CAD build for the part. Positions are in the model's coordinates, mm. Give positions to 0.01 mm unless a question says otherwise; leave off trailing zeros. Order: outer loops, then holes, each group sorted by start corner. A loop starts at its lowest first (then second) coordinate and runs counter-clockwise, first axis right, second up.
from build123d import *

# Parameters (mm, degrees)
FLOOR_MOUNT_AND_JOINT_HOLES_PROFILE_R   = 2.75
FLOOR_MOUNT_AND_JOINT_HOLES_PROFILE_R_2 = 1.75
FLOOR_MOUNT_AND_JOINT_HOLES_PROFILE_R_3 = 2.25
FLOOR_MOUNT_AND_JOINT_HOLES_PROFILE_R_4 = 2.2
FLOOR_MOUNT_AND_JOINT_HOLES_DEPTH       = 1


with BuildPart() as part:
    # Floor, mount and joint holes profile → Floor, mount and joint holes (new body)
    with BuildSketch(Plane.XY):
        Polygon((-140, -143), (-94, -143), (-94, -104), (93, -104), (93, -143), (103, -143), (103, 143), (93, 143), (93, 104), (-94, 104), (-94, 143), (-140, 143), align=None)
        with Locations((-90, -91)):
            Circle(FLOOR_MOUNT_AND_JOINT_HOLES_PROFILE_R, mode=Mode.SUBTRACT)
        with Locations((-90, 91)):
            Circle(FLOOR_MOUNT_AND_JOINT_HOLES_PROFILE_R, mode=Mode.SUBTRACT)
        with Locations((-31, -91)):
            Circle(FLOOR_MOUNT_AND_JOINT_HOLES_PROFILE_R, mode=Mode.SUBTRACT)
        with Locations((-31, 91)):
            Circle(FLOOR_MOUNT_AND_JOINT_HOLES_PROFILE_R, mode=Mode.SUBTRACT)
        with Locations((31, -91)):
            Circle(FLOOR_MOUNT_AND_JOINT_HOLES_PROFILE_R, mode=Mode.SUBTRACT)
        with Locations((31, 91)):
            Circle(FLOOR_MOUNT_AND_JOINT_HOLES_PROFILE_R, mode=Mode.SUBTRACT)
        with Locations((90, -91)):
            Circle(FLOOR_MOUNT_AND_JOINT_HOLES_PROFILE_R, mode=Mode.SUBTRACT)
        with Locations((90, 91)):
            Circle(FLOOR_MOUNT_AND_JOINT_HOLES_PROFILE_R, mode=Mode.SUBTRACT)
        with Locations((-136.5, -108)):
            Circle(FLOOR_MOUNT_AND_JOINT_HOLES_PROFILE_R_2, mode=Mode.SUBTRACT)
        with Locations((-136.5, -17)):
            Circle(FLOOR_MOUNT_AND_JOINT_HOLES_PROFILE_R_2, mode=Mode.SUBTRACT)
        with Locations((-136.5, 17)):
            Circle(FLOOR_MOUNT_AND_JOINT_HOLES_PROFILE_R_2, mode=Mode.SUBTRACT)
        with Locations((-136.5, 108)):
            Circle(FLOOR_MOUNT_AND_JOINT_HOLES_PROFILE_R_2, mode=Mode.SUBTRACT)
        with Locations((-100.5, -108)):
            Circle(FLOOR_MOUNT_AND_JOINT_HOLES_PROFILE_R_2, mode=Mode.SUBTRACT)
        with Locations((-100.5, -17)):
            Circle(FLOOR_MOUNT_AND_JOINT_HOLES_PROFILE_R_2, mode=Mode.SUBTRACT)
        with Locations((-100.5, 17)):
            Circle(FLOOR_MOUNT_AND_JOINT_HOLES_PROFILE_R_2, mode=Mode.SUBTRACT)
        with Locations((-100.5, 108)):
            Circle(FLOOR_MOUNT_AND_JOINT_HOLES_PROFILE_R_2, mode=Mode.SUBTRACT)
        with Locations((-92.5, -46)):
            Circle(FLOOR_MOUNT_AND_JOINT_HOLES_PROFILE_R_3, mode=Mode.SUBTRACT)
        with Locations((-92.5, 46)):
            Circle(FLOOR_MOUNT_AND_JOINT_HOLES_PROFILE_R_3, mode=Mode.SUBTRACT)
        with Locations((-43.5, -46)):
            Circle(FLOOR_MOUNT_AND_JOINT_HOLES_PROFILE_R_3, mode=Mode.SUBTRACT)
        with Locations((-43.5, 46)):
            Circle(FLOOR_MOUNT_AND_JOINT_HOLES_PROFILE_R_3, mode=Mode.SUBTRACT)
        with Locations((-30.5, -46)):
            Circle(FLOOR_MOUNT_AND_JOINT_HOLES_PROFILE_R_3, mode=Mode.SUBTRACT)
        with Locations((-30.5, 46)):
            Circle(FLOOR_MOUNT_AND_JOINT_HOLES_PROFILE_R_3, mode=Mode.SUBTRACT)
        with Locations((18.5, -46)):
            Circle(FLOOR_MOUNT_AND_JOINT_HOLES_PROFILE_R_3, mode=Mode.SUBTRACT)
        with Locations((18.5, 46)):
            Circle(FLOOR_MOUNT_AND_JOINT_HOLES_PROFILE_R_3, mode=Mode.SUBTRACT)
        with Locations((31.5, -46)):
            Circle(FLOOR_MOUNT_AND_JOINT_HOLES_PROFILE_R_3, mode=Mode.SUBTRACT)
        with Locations((31.5, 46)):
            Circle(FLOOR_MOUNT_AND_JOINT_HOLES_PROFILE_R_3, mode=Mode.SUBTRACT)
        with Locations((80.5, -46)):
            Circle(FLOOR_MOUNT_AND_JOINT_HOLES_PROFILE_R_3, mode=Mode.SUBTRACT)
        with Locations((80.5, 46)):
            Circle(FLOOR_MOUNT_AND_JOINT_HOLES_PROFILE_R_3, mode=Mode.SUBTRACT)
        with Locations((-117, -135)):
            Circle(FLOOR_MOUNT_AND_JOINT_HOLES_PROFILE_R, mode=Mode.SUBTRACT)
        with Locations((-117, 135)):
            Circle(FLOOR_MOUNT_AND_JOINT_HOLES_PROFILE_R, mode=Mode.SUBTRACT)
        with Locations((98, -135)):
            Circle(FLOOR_MOUNT_AND_JOINT_HOLES_PROFILE_R, mode=Mode.SUBTRACT)
        with Locations((98, 135)):
            Circle(FLOOR_MOUNT_AND_JOINT_HOLES_PROFILE_R, mode=Mode.SUBTRACT)
        with Locations((98.5, -105)):
            Circle(FLOOR_MOUNT_AND_JOINT_HOLES_PROFILE_R, mode=Mode.SUBTRACT)
        with Locations((98.5, -55)):
            Circle(FLOOR_MOUNT_AND_JOINT_HOLES_PROFILE_R, mode=Mode.SUBTRACT)
        with Locations((98.5, 0)):
            Circle(FLOOR_MOUNT_AND_JOINT_HOLES_PROFILE_R, mode=Mode.SUBTRACT)
        with Locations((98.5, 55)):
            Circle(FLOOR_MOUNT_AND_JOINT_HOLES_PROFILE_R, mode=Mode.SUBTRACT)
        with Locations((98.5, 105)):
            Circle(FLOOR_MOUNT_AND_JOINT_HOLES_PROFILE_R, mode=Mode.SUBTRACT)
        with Locations((-134, -130)):
            Circle(FLOOR_MOUNT_AND_JOINT_HOLES_PROFILE_R_4, mode=Mode.SUBTRACT)
        with Locations((-134, 0)):
            Circle(FLOOR_MOUNT_AND_JOINT_HOLES_PROFILE_R_4, mode=Mode.SUBTRACT)
        with Locations((-134, 130)):
            Circle(FLOOR_MOUNT_AND_JOINT_HOLES_PROFILE_R_4, mode=Mode.SUBTRACT)
        with Locations((-37, -81)):
            Circle(FLOOR_MOUNT_AND_JOINT_HOLES_PROFILE_R_4, mode=Mode.SUBTRACT)
        with Locations((-37, 81)):
            Circle(FLOOR_MOUNT_AND_JOINT_HOLES_PROFILE_R_4, mode=Mode.SUBTRACT)
        with Locations((30, -81)):
            Circle(FLOOR_MOUNT_AND_JOINT_HOLES_PROFILE_R_4, mode=Mode.SUBTRACT)
        with Locations((30, 81)):
            Circle(FLOOR_MOUNT_AND_JOINT_HOLES_PROFILE_R_4, mode=Mode.SUBTRACT)
        with Locations((-132, -115)):
            Circle(FLOOR_MOUNT_AND_JOINT_HOLES_PROFILE_R_2, mode=Mode.SUBTRACT)
        with Locations((-132, -5)):
            Circle(FLOOR_MOUNT_AND_JOINT_HOLES_PROFILE_R_2, mode=Mode.SUBTRACT)
        with Locations((-132, 5)):
            Circle(FLOOR_MOUNT_AND_JOINT_HOLES_PROFILE_R_2, mode=Mode.SUBTRACT)
        with Locations((-132, 115)):
            Circle(FLOOR_MOUNT_AND_JOINT_HOLES_PROFILE_R_2, mode=Mode.SUBTRACT)
        with Locations((-100, -115)):
            Circle(FLOOR_MOUNT_AND_JOINT_HOLES_PROFILE_R_2, mode=Mode.SUBTRACT)
        with Locations((-100, -5)):
            Circle(FLOOR_MOUNT_AND_JOINT_HOLES_PROFILE_R_2, mode=Mode.SUBTRACT)
        with Locations((-100, 5)):
            Circle(FLOOR_MOUNT_AND_JOINT_HOLES_PROFILE_R_2, mode=Mode.SUBTRACT)
        with Locations((-100, 115)):
            Circle(FLOOR_MOUNT_AND_JOINT_HOLES_PROFILE_R_2, mode=Mode.SUBTRACT)
    extrude(amount=FLOOR_MOUNT_AND_JOINT_HOLES_DEPTH)


solid = part.part
1. Saw through at A-A on z = 0.4. State how many separate pieces and enclosed holes the cut face has, plus the area to 3 significant figures.
2. Saw through at B-B on x = 56. Give the cut face in (y, z), plus the area to 3 significant figures.
3. Wall check: line 1 (Y direction, x = 81, z = 0.95); line 2 (X direction, y = -90.5, z = 0.8); line 3 (Y direction, x = -136.5, z = 0.25). Give the ranges that are in metal, low to high.
4. Pin check, flat tip, straight feed: P1, Ø5, axis at x = -77.5, y = -45, coming from the -Z side. Stop position of the tip, or through.
Reported:
1. separate pieces: 1
1. enclosed holes: 52
1. area: 54,100 mm2
2. outline: (-104, 0) - (104, 0) - (104, 1) - (-104, 1) - close
2. area: 208 mm2
3. line 1: y = -104 to -48.19, -43.81 to 43.81, 48.19 to 104
3. line 2: x = -140 to -92.7, -87.3 to -33.7, -28.3 to 28.3, 33.7 to 87.3, 92.7 to 103
3. line 3: y = -143 to -109.75, -106.25 to -18.75, -15.25 to 15.25, 18.75 to 106.25, 109.75 to 143
4. P1: stops at z = 0
